Input: part model. Units: mm. Frame: model coordinates. Face numbers are marked on the shaded views. A direction names the side the tool comes from. Coordinates: 2 decimals unless noted, no trailing zeros. Loops run counter-clockwise (first coordinate to the right, second up) from the corner with the lowest first, then second, coordinate; pieces in that order, holes last. Notation, with made-up numbers: (19.5, 27.5) - (55.5, 27.5) arc R22 cw to (55.5, 61.5) - close; hole circle Ø1 at (-36.5, 50). An arc over 180 degrees is marked (long way). Write item = value, one per line. Start each with the question number.
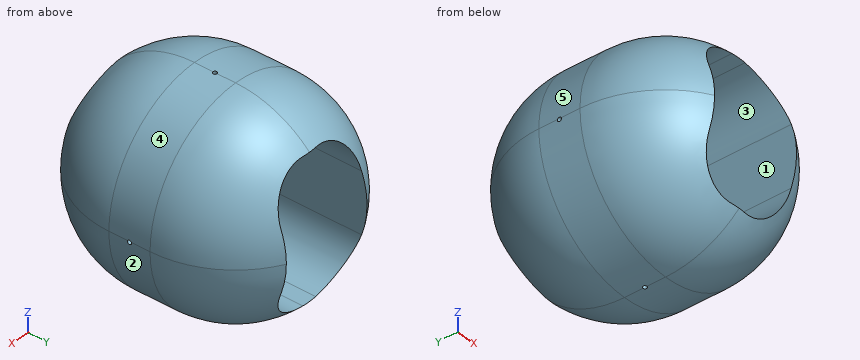
from build123d import *

# Parameters (mm, degrees)
F0_W          = 127
F0_H          = 127
F1_DEPTH      = 152.4
F2_R          = 63.49999
F3_W          = 60.3535668924
F3_H          = 88.5923877358
F4_DEPTH      = 187.706
F5_R          = 25.4
F6_R          = 1.27
F7_DEPTH      = 62.9846544394
F7_DEPTH_BACK = 95.758
F8_R          = 1.27
F9_DEPTH      = 78.9673156079
F9_DEPTH_BACK = 48.0346845921


# Not quite as in the source:
# - a fillet or chamfer is up to 0.001 mm smaller than in the source, because OpenCascade refuses the exact size


with BuildPart() as f1:
    # F0 (on Front) → F1 (new body)
    with BuildSketch(Plane.XZ):
        with Locations((15.4663155079, 0.5163455606)):
            Rectangle(F0_W, F0_H)
    extrude(amount=F1_DEPTH)

    # F2 (radius 63.5 in the source; OpenCascade refuses exactly that, so slightly less here)
    f2_edges = [f1.edges().sort_by_distance(p)[0] for p in [
        (-48.033684, -76.2, 64.016346),
        (-48.033684, -152.4, 0.516346),
        (15.466316, -152.4, 64.016346),
        (78.966316, -152.4, 0.516346),
        (78.966316, -76.2, 64.016346),
        (78.966316, 0, 0.516346),
        (15.466316, 0, -62.983654),
        (78.966316, -76.2, -62.983654),
        (-48.033684, -76.2, -62.983654),
        (-48.033684, 0, 0.516346),
        (15.466316, -152.4, -62.983654),
        (15.466316, 0, 64.016346),
    ]]
    fillet(f2_edges, radius=F2_R)

    # F3 (on Front) → F4 (cut)
    with BuildSketch(Plane.XZ):
        with Locations((15.0872929953, 0.415276736)):
            Rectangle(F3_W, F3_H)
    extrude(amount=F4_DEPTH, mode=Mode.SUBTRACT)

    # F5
    f5_edges = [f1.edges().sort_by_distance(p)[0] for p in [
        (45.264076, -76.2, -43.880917),
        (45.264076, -76.2, 44.711471),
        (-15.08949, -76.2, 44.711471),
        (-15.08949, -76.2, -43.880917),
    ]]
    fillet(f5_edges, radius=F5_R)

    # F6 (on Top) → F7 (cut, two sides)
    with BuildSketch(Plane.XY) as f7_sk:
        with Locations((15.4663155079, -76.2)):
            Circle(F6_R)
    extrude(amount=-F7_DEPTH, mode=Mode.SUBTRACT)
    extrude(f7_sk.sketch, amount=F7_DEPTH_BACK, mode=Mode.SUBTRACT)

    # F8 (on Right) → F9 (cut, two sides)
    with BuildSketch(Plane.YZ) as f9_sk:
        with Locations((-76.2, 0)):
            Circle(F8_R)
    extrude(amount=F9_DEPTH, mode=Mode.SUBTRACT)
    extrude(f9_sk.sketch, amount=-F9_DEPTH_BACK, mode=Mode.SUBTRACT)


solid = f1.part
Item 1: Pin query (flat end, axial travel): pin 1 (4 mm diameter, centred on y = -80, z = 37.5, fed in from -X); pin 2 (3 mm diameter, centred on x = 4.5, y = -67.5, fed in from +Z); pin 3 (8 mm diameter, centred on y = -81.5, z = -16.5, fed in from -X). Return the tip coordinate at first contact, or that it passes through.
Item 2: Cut plane A-A on z = 4. Return loops of the section in (x, y).
Item 3: Access query for the marked faces 1 and 2. Directions: +Z, -Z, +X, -X, +Y, -Y. A direction counts if a zero-diameter tool reaches every point of the face in a straight line with its end or side. Return the directions, or none.
Item 4: Pull-direction query (X, two-part tool) for the marked faces 3, 4 and 5; classes: pulls with the +X half, pulls with the -X half, needs draft (parallel to the pull), parting line crosses it, or undercut.
Item 5: Ray query, line 1 (Z direction, x = 7.5, y = -117.5); line 2 (Y direction, x = -21, z = 0); line 3 (Z direction, x = -10, y = -89). Return the intervals inside material, ascending.
Item 6: Cut plane B-B on x = 1. Return loops of the section in (y, z).
Recorded:
q1.pin_1 = -37.53
q1.pin_2 = 63.31
q1.pin_3 = -46.69
q2.outline = (-47.94, -88.9) arc R63.4 ccw to (-15.09, -144.46) - (-15.09, -7.94) arc R63.4 ccw to (-47.94, -63.5) - close; (45.26, -144.87) arc R63.4 ccw to (78.87, -88.9) - (78.87, -63.5) arc R63.4 ccw to (45.26, -7.53) - close
q3.face_1 = +Y, -Y
q3.face_2 = -Z, +X, +Y, -Y
q4.face_3 = undercut
q4.face_4 = pulls with the +X half
q4.face_5 = pulls with the -X half
q5.line_1 = -55.62 to -43.72, 44.56 to 56.65
q5.line_2 = -140.88 to -77.47, -74.93 to -11.52
q5.line_3 = -57.65 to -33.73, 34.56 to 58.69
q6.outline = (-133.88, 42.94) - (-18.52, 42.94) arc R61.83 ccw to (-63.5, 62.35) - (-88.9, 62.35) arc R61.83 ccw to start; (-133.69, -42.11) arc R61.83 ccw to (-88.9, -61.31) - (-63.5, -61.31) arc R61.83 ccw to (-18.71, -42.11) - close
